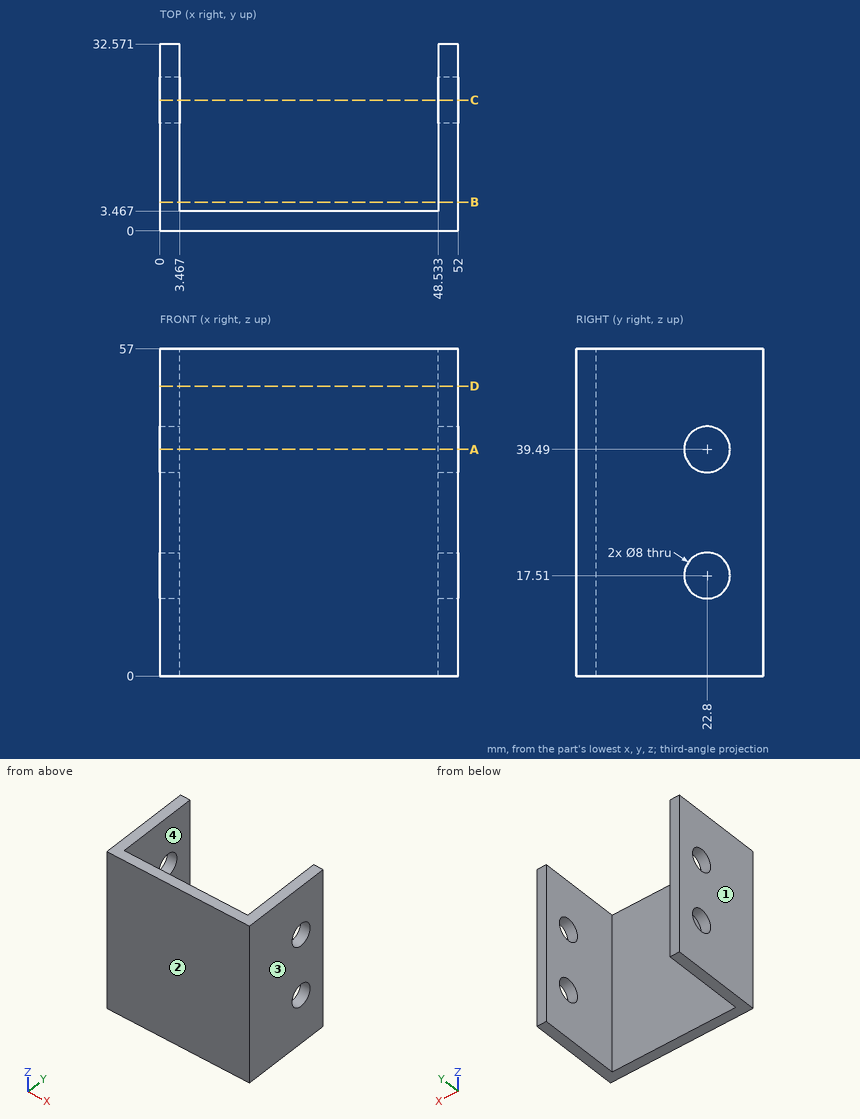
Answer from the drawing. Dimensions are ordinates in mm from the lowest x, y and z of the part. Round coordinates to 2 decimals unless told otherwise and drop trailing zeros. Loops run counter-clockwise (first coordinate to the right, second up) from the corner with the lowest first, then second, coordinate; pieces in that order, holes last. Notation, with made-up numbers: (-0.5, -6) - (52.5, -6) arc R18 ccw to (52.5, 10) - close; hole circle Ø7 at (26.5, -4). An arc over 180 degrees is marked (long way). Return JSON: item names as keys, results as strings. Group by question number.
1. The part is cut by section C-C on y = 22.8. Determine the outline of the cut face in (x, z), then the cut area to 3 significant figures.
2. This flat-tipped pin is pushed along its axis until it touches: P1, Ø14.5, axis at y = 12, z = 29, coming from the -X side. Where does it stop, or does it pass through?
3. The part is cut by section D-D on z = 50.5. Determine the outline of the cut face in (x, y).
4. The part is cut by section B-B on y = 5. Determine the outline of the cut face in (x, z), then the cut area to 3 significant figures.
5. Consider probe 1 along Z at (x, y) = (0.9, 22.8); probe 2 along X at (y, z) = (21, 5.5); probe 3 along Y at (x, z) = (1.6, 17.51). Determine where each line is inside the solid, lowest interval first.
6. The part is cut by section A-A on z = 39.49. Determine the outline of the cut face in (x, y).
7. The mould has two halves that part along X. Classify the marked faces 1, 2, 3 and 4: pulls with the +X half, pulls with the -X half, needs draft (parallel to the pull), parting line crosses it, or undercut.
Resolved:
{
 "1": {"outline": "(0, 0) - (3.47, 0) - (3.47, 13.51) - (0, 13.51) - close; (0, 21.51) - (3.47, 21.51) - (3.47, 35.49) - (0, 35.49) - close; (0, 43.49) - (3.47, 43.49) - (3.47, 57) - (0, 57) - close; (48.53, 0) - (52, 0) - (52, 13.51) - (48.53, 13.51) - close; (48.53, 21.51) - (52, 21.51) - (52, 35.49) - (48.53, 35.49) - close; (48.53, 43.49) - (52, 43.49) - (52, 57) - (48.53, 57) - close", "area": "284 mm²"},
 "2": {"P1": "stops at x = 0"},
 "3": {"outline": "(0, 0) - (52, 0) - (52, 32.57) - (48.53, 32.57) - (48.53, 3.47) - (3.47, 3.47) - (3.47, 32.57) - (0, 32.57) - close"},
 "4": {"outline": "(0, 0) - (3.47, 0) - (3.47, 57) - (0, 57) - close; (48.53, 0) - (52, 0) - (52, 57) - (48.53, 57) - close", "area": "395 mm²"},
 "5": {"probe 1": "z = 0 to 13.51, 21.51 to 35.49, 43.49 to 57", "probe 2": "x = 0 to 3.47, 48.53 to 52", "probe 3": "y = 0 to 18.8, 26.8 to 32.57"},
 "6": {"outline": "(0, 0) - (52, 0) - (52, 18.8) - (48.53, 18.8) - (48.53, 3.47) - (3.47, 3.47) - (3.47, 18.8) - (0, 18.8) - close; (0, 26.8) - (3.47, 26.8) - (3.47, 32.57) - (0, 32.57) - close; (48.53, 26.8) - (52, 26.8) - (52, 32.57) - (48.53, 32.57) - close"},
 "7": {"face 1": "pulls with the -X half", "face 2": "needs draft", "face 3": "pulls with the +X half", "face 4": "undercut"}
}
